```python
from build123d import *

# Parameters (mm, degrees)
P_IDAT_VYSUNUT_M1_DEPTH  = 15
ODEBRAT_VYSUNUT_M1_DEPTH = 82.091450741
LINPOLE1_COUNT           = 5
LINPOLE1_PITCH           = 10
SKICA3_W                 = 20
SKICA3_H                 = 5
P_IDAT_VYSUNUT_M2_DEPTH  = 11.5
ZKOSEN_1_SIZE            = 1
ZAOBLIT1_R               = 1
SKICA4_W                 = 20
SKICA4_H                 = 5
P_IDAT_VYSUNUT_M3_DEPTH  = 6.5
ZAOBLIT2_R               = 2
ZAOBLIT3_R               = 3


with BuildPart() as part:
    # Skica1 → Přidat vysunutím1 (new body)
    with BuildSketch(Plane.XY):
        with BuildLine():
            Line((-2.25, 79.062148865), (-10, 79.062148865))
            Line((-10, 79.062148865), (-10, 0))
            Line((-10, 0), (10, 0))
            Line((10, 0), (10, 79.062148865))
            Line((10, 79.062148865), (2.25, 79.062148865))
            ThreePointArc((2.25, 79.062148865), (1.268413323, 78.253166128), (1.875, 77.135124054))
            ThreePointArc((1.875, 77.135124054), (0, 67.5), (-1.875, 77.135124054))
            ThreePointArc((-1.875, 77.135124054), (-1.268413323, 78.253166128), (-2.25, 79.062148865))
        make_face()
    extrude(amount=P_IDAT_VYSUNUT_M1_DEPTH)

    # Skica2 → Odebrat vysunutím1 (cut, through all)
    with BuildSketch(Plane.XY.offset(15)):
        with BuildLine():
            Line((-8, 56), (-8, 59))
            ThreePointArc((-8, 59), (-6.5, 60.5), (-5, 59))
            Line((-5, 59), (-5, 56))
            ThreePointArc((-5, 56), (-6.5, 54.5), (-8, 56))
        make_face()
        with BuildLine():
            Line((5, 56), (5, 59))
            ThreePointArc((5, 59), (6.5, 60.5), (8, 59))
            Line((8, 59), (8, 56))
            ThreePointArc((8, 56), (6.5, 54.5), (5, 56))
        make_face()
    odebrat_vysunut_m1 = extrude(amount=-ODEBRAT_VYSUNUT_M1_DEPTH, mode=Mode.SUBTRACT)

    # LinPole1: Odebrat vysunutím1 ×5
    with Locations(*[(0, -i * LINPOLE1_PITCH, 0) for i in range(1, LINPOLE1_COUNT)]):
        add(odebrat_vysunut_m1, mode=Mode.SUBTRACT)

    # Skica3 → Přidat vysunutím2 (add)
    with BuildSketch(Plane.XZ):
        with Locations((0, 2.5)):
            Rectangle(SKICA3_W, SKICA3_H)
    extrude(amount=P_IDAT_VYSUNUT_M2_DEPTH)

    # Zkosení1
    zkosen_1_edges = [part.edges().sort_by_distance(p)[0] for p in [
        (-10, -11.5, 2.5),
        (10, -11.5, 2.5),
    ]]
    chamfer(zkosen_1_edges, length=ZKOSEN_1_SIZE)

    # Zaoblit1
    zaoblit1_edges = [part.edges().sort_by_distance(p)[0] for p in [
        (10, 79.062148865, 7.5),
        (-10, 79.062148865, 7.5),
    ]]
    fillet(zaoblit1_edges, radius=ZAOBLIT1_R)

    # Skica4 → Přidat vysunutím3 (add)
    with BuildSketch(Plane.XY.offset(15)):
        with Locations((0, 2.5)):
            Rectangle(SKICA4_W, SKICA4_H)
    extrude(amount=P_IDAT_VYSUNUT_M3_DEPTH)

    # Zaoblit2
    zaoblit2_edges = [part.edges().sort_by_distance(p)[0] for p in [
        (-10, 2.5, 21.5),
        (10, 2.5, 21.5),
    ]]
    fillet(zaoblit2_edges, radius=ZAOBLIT2_R)

    # Zaoblit3
    zaoblit3_edges = [part.edges().sort_by_distance(p)[0] for p in [
        (0, 5, 15),
    ]]
    fillet(zaoblit3_edges, radius=ZAOBLIT3_R)


solid = part.part
```
The model under review builds one solid part; all positions refer to its coordinate system, in mm. Round coordinates to 2 decimals unless told otherwise and drop trailing zeros. Order: outer loops, then holes, each group sorted by start corner. A loop starts at its lowest first (then second) coordinate and runs counter-clockwise, first axis right, second up. Notation, with made-up numbers: (-4.75, 16.5) -> (32.25, 16.5) arc R21 cw to (32.25, 20.5) -> close; hole circle Ø4 at (88.5, -27.75). An arc over 180 degrees is marked (long way). One line per item, written item: value. Start each with the question number.
Q1. Take a section at A-A (x = 6.5). Count the separate pieces of the cut face and the enclosed holes in it, and give its area (3 significant figures).
Q2. Wall thickness on line 1 (X direction, y = 47.5, z = 2); line 2 (X direction, y = 72.5, z = 4.25); line 3 (Y direction, x = 5.5, z = 13): over which ranges is each line inside the solid? List them lowest first.
Q3. Mouldability with a two-part tool opening along Y and no side actions: class faces 1 (the face through (9.43, 2.54, 20.9)), 2 (the face through (8, 48, 8)), 3 (the face through (0.14, 5.86, 15.9)) as released by +Y, released by -Y, zero draft, split by the parting line, or undercut.
Q4. Take a section at B-B (y = 70.5). Write out the cut boundary in (x, z), and give its area (3 significant figures).
Q5. Clearance check with flat-ended pins moving along their axes: pin 1 Ø2 at (x, z) = (-4.5, 9) entering from -Y; pin 2 Ø8 at (x, y) = (0.5, 28.5) entering from +Z; pin 3 Ø10 at (y, z) = (19.5, 19) entering from +X; pin 4 Ø3 at (x, z) = (2.5, 19) entering from +Y. State where each tip first meets the part, or that it passes through.
Q6. Take a section at C-C (y = 10). Write out the cut boundary in (x, z), and give its area (3 significant figures).
Reported:
1. separate pieces: 6
1. enclosed holes: 0
1. area: 828 mm2
2. line 1: x = -10 to -8, -5 to 5, 8 to 10
2. line 2: x = -10 to -5, 5 to 10
2. line 3: y = 0 to 14.88, 20.12 to 24.88, 30.12 to 34.88, 40.12 to 44.88, 50.12 to 54.88, 60.12 to 79.06
3. face 1: zero draft
3. face 2: undercut
3. face 3: released by +Y
4. outline: (-10, 0) -> (-4.58, 0) -> (-4.58, 15) -> (-10, 15) -> close; (4.58, 0) -> (10, 0) -> (10, 15) -> (4.58, 15) -> close
4. area: 163 mm2
5. pin 1: stops at y = 0
5. pin 2: stops at z = 15
5. pin 3: stops at x = 10
5. pin 4: stops at y = 5.04
6. outline: (-10, 0) -> (10, 0) -> (10, 15) -> (-10, 15) -> close
6. area: 300 mm2
